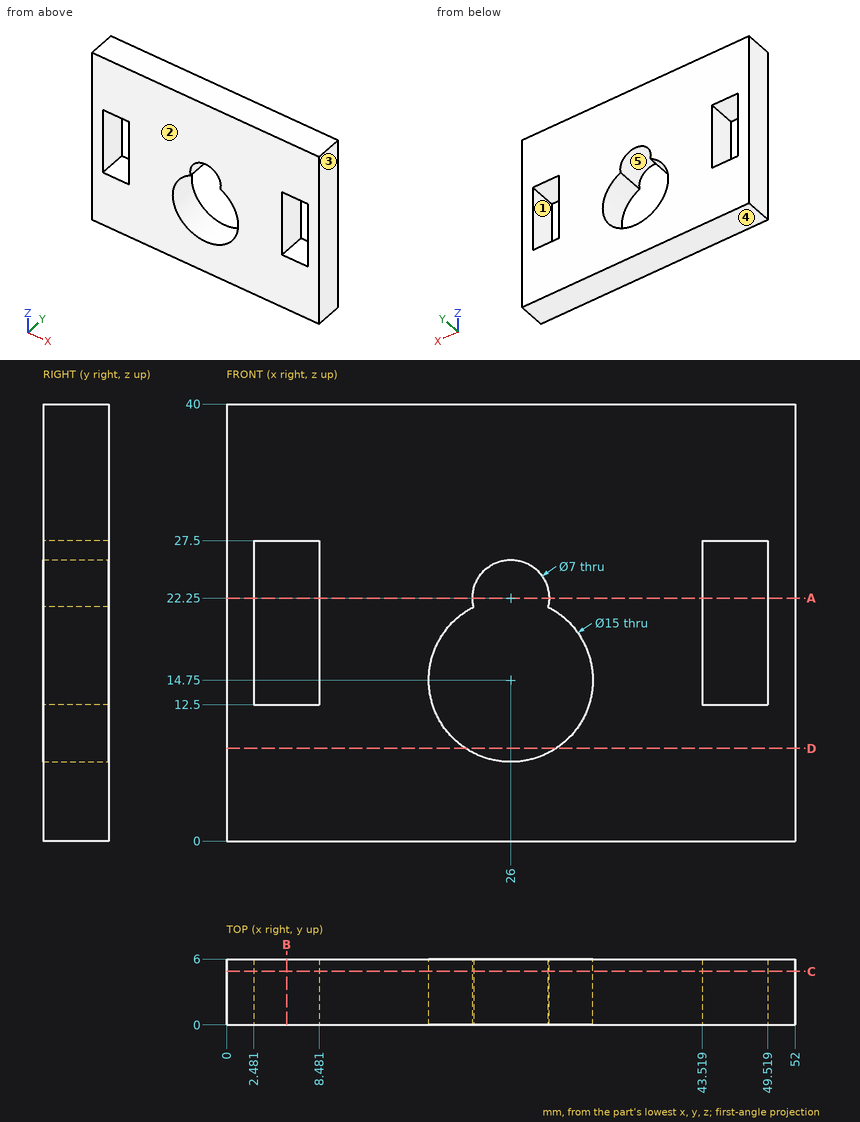
The figure shows three views and two pictorial views of one solid part (mm, origin at its lowest corner). Answer the questions. A direction names the side the tool comes from. Round coordinates to 2 decimals unless told otherwise and drop trailing zeros. Order: outer loops, then holes, each group sorted by start corner. A loop starts at its lowest first (then second) coordinate and runs counter-clockwise, first axis right, second up. Notation, with made-up numbers: M 19,84 L 41,84 A13 ccw 41,102 Z; hole C 67.25,37 d1. An arc over 180 degrees is marked long. Put each result on its own line as item: value. Start each with the question number.
Q1. Section B-B, the plane x = 5.5 is taken. Write down the section's boundary in (y, z).
Q2. Straight lines are drawn through the part: L1, parallel to X at y = 5.65, z = 22; L2, parallel to X at y = 2.45, z = 14.75; L3, parallel to Z at x = 26, y = 2.7. For each, find the intervals that lie inside material, in ascending order. Write a range as [from, to].
Q3. For a pull along Z with two mould halves and no side action, classify the marked faces 3, 4 and 5 as pulls with the +Z half, pulls with the -Z half, needs draft (parallel to the pull), parting line crosses it, or undercut.
Q4. Flat-ended cylindrical pins translate along their axes: pin 1 (19.5 mm diameter, centred on x = 26, z = 14.75, fed in from +Y); pin 2 (2 mm diameter, centred on x = 21.5, z = 13, fed in from +Y). Find the tip coordinate at first contact, or state that the pin passes through.
Q5. A tool of negligible diameter and unlimited length cuts with its end or side. For the marked faces 1 and 2, from which of +Z, -Z, +X, -X, +Y, -Y can it reach the whole face along a straight path? Write none if from no direction.
Q6. Section D-D, the plane z = 8.5 is taken. Write down the section's boundary in (x, y), and give its area (3 significant figures).
Q7. Section A-A, the plane z = 22.25 is taken. Write down the section's boundary in (x, y).
Q8. Section C-C, the plane y = 4.9 is taken. Write down the section's boundary in (x, z), and give its area (3 significant figures).
Findings below:
1. outline: M 0,0 L 6,0 L 6,12.5 L 0,12.5 Z; M 0,27.5 L 6,27.5 L 6,40 L 0,40 Z
2. L1: x = [0, 2.48], [8.48, 22.51], [29.49, 43.52], [49.52, 52]
2. L2: x = [0, 2.48], [8.48, 18.5], [33.5, 43.52], [49.52, 52]
2. L3: z = [0, 7.25], [25.75, 40]
3. face 3: needs draft
3. face 4: pulls with the -Z half
3. face 5: undercut
4. pin 1: stops at y = 6
4. pin 2: passes through
5. face 1: +Y, -Y
5. face 2: +Z, -Z, +X, -X, -Y
6. outline: M 0,0 L 21.85,0 L 21.85,6 L 0,6 Z; M 30.15,0 L 52,0 L 52,6 L 30.15,6 Z
6. area: 262 mm^2
7. outline: M 0,0 L 2.48,0 L 2.48,6 L 0,6 Z; M 8.48,0 L 22.5,0 L 22.5,6 L 8.48,6 Z; M 29.5,0 L 43.52,0 L 43.52,6 L 29.5,6 Z; M 49.52,0 L 52,0 L 52,6 L 49.52,6 Z
8. outline: M 0,0 L 52,0 L 52,40 L 0,40 Z; hole M 2.48,12.5 L 8.48,12.5 L 8.48,27.5 L 2.48,27.5 Z; hole M 22.6,21.43 A7.5 ccw long 29.4,21.43 A3.5 ccw long Z; hole M 43.52,12.5 L 49.52,12.5 L 49.52,27.5 L 43.52,27.5 Z
8. area: 1,700 mm^2
